Could you check a few things on this model? Use its own coordinates, in mm. Give positions to 0.01 mm unless a question says otherwise; leave off trailing zeros. Write each question's results on one line, items separated by ' | '.
Autodesk Inventor part; units mm, degrees
ref_plane "YZ Plane" through (0, 0, 0) normal (1, 0, 0) x (0, 1, 0)
ref_plane "XZ Plane" through (0, 0, 0) normal (0, 1, 0) x (-1, 0, 0)
ref_plane "XY Plane" through (0, 0, 0) normal (0, 0, 1) x (1, 0, 0)
sketch "Boceto1" plane through (0, 0, 0) normal (1, 0, 0) x (0, 1, 0)
  line L0 (0, 0) -> (0, 125)
  line L1 (0, 0) -> (125, 0) construction
  line L2 (0, 0) -> (0, -125)
  line L3 (0, 0) -> (125, 0) construction
  line L4 (0, 0) -> (-20, 0)
  line L5 (0, 0) -> (20, 0) construction
  line L6 (0, 0) -> (500, 0) construction
  line L7 (0, 0) -> (-20, 0)
  line L8 (0, 0) -> (20, 0) construction
  line L9 (0, 0) -> (0, -246.4363)
  line L10 (0, 0) -> (246.4363, 0) construction
  line L11 (0, 0) -> (0, 250)
  line L12 (0, 0) -> (250, 0) construction
  arc A0 (0, 250) -> (0, -246.4363) centre (1530.2267, 1.7819) ccw
  line L13 (0, 125) -> (-100, 125)
  line L14 (0, 125) -> (100, 125) construction
  line L15 (0, 250) -> (-5, 250)
  line L16 (0, 250) -> (5, 250) construction
  line L17 (0, -246.4363) -> (-5, -246.4363)
  line L18 (-20, 0) -> (-23, 0)
  line L19 (-20, 0) -> (-17, 0) construction
  line L20 (-20, 0) -> (-25, 0)
  line L21 (-20, 0) -> (-15, 0) construction
  arc A1 (-5, 250) -> (-5, -246.4363) centre (1525.2267, 1.7819) ccw
  point P0 (-20.0963, 125)
  point P1 (-15.0963, 125)
  dimension "d14" = 100
  dimension "d15" = 180
  dimension "d16" = 5
  dimension "d17" = 180
  dimension "d18" = 5
  dimension "d19" = 3
  dimension "d20" = 180
  dimension "d21" = 5
  dimension "d22" = 180
revolve "Revolución1" add sketch "Boceto1" angle 90 about axis through (0, -20, 0) along (0, -1, 0) contours L18 L20 A1 L13 A0
fillet "Empalme1" radius 2 2 edges at (-88.3883, -15.0963, 88.3883) (-88.3883, -20.0963, 88.3883)
Q1. I need wall thicknesses on line 1 along Y through (x, z) = (-88.5, 76); line 2 along Y through (x, z) = (-25, 46.5); line 3 along Z through (x, y) = (-64, -20). Which ranges of each line are inside material? Lowest first, please.
Here are the results:
line 1: y = -20.74 to -15.74 | line 2: y = -24.16 to -19.16 | line 3: z = 0 to 106.17
Q2. I'm going to push flat-ended pins straight in: pin 1 Ø6 at (x, z) = (-59.5, 85) entering from -Y; pin 2 Ø2 at (x, z) = (-39, 61.5) entering from +Y; pin 3 Ø5 at (y, z) = (-20.5, 73) entering from -X. Where does each tip first touch, or does it pass through?
Here are the results:
pin 1: stops at y = -21.84 | pin 2: stops at y = -18.33 | pin 3: stops at x = -102.7
Q3. Thinking about a two-plate mould opening in X: for faces 1 (the flat face through (0, -21, 63)), 2 (the flat face through (-63, -21, 0)), 3 (the cylindrical face through (-87.411, -17.761, 89.355)), which applies, +X half, -X half, draft (parallel to the pull), parting line (faces both ways), or undercut?
Here are the results:
face 1: +X half | face 2: draft | face 3: -X half
